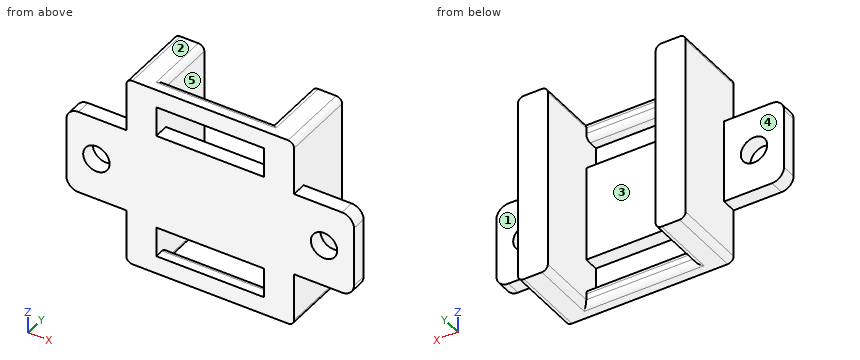
from build123d import *

# Parameters (mm, degrees)
SKETCH1_W           = 28
SKETCH1_H           = 32
BOSS_EXTRUDE1_DEPTH = 2.5
BOSS_EXTRUDE3_DEPTH = 10
SKETCH3_W           = 18
SKETCH3_H           = 8
CUT_EXTRUDE1_DEPTH  = 2.5
SKETCH4_W           = 10
SKETCH4_H           = 14
SKETCH4_R           = 2.2
BOSS_EXTRUDE4_DEPTH = 2.5
FILLET1_R           = 2
FILLET2_R           = 1
SKETCH5_W           = 24.202572411
SKETCH5_H           = 3
SKETCH5_W_2         = 23.282926667
BOSS_EXTRUDE5_DEPTH = 2.5
FILLET3_R           = 1


with BuildPart() as part:
    # Sketch1 → Boss-Extrude1 (new body)
    with BuildSketch(Plane(origin=(0, 0, 0), x_dir=(1, 0, 0), z_dir=(0, 1, 0))):
        with Locations((14, 16)):
            Rectangle(SKETCH1_W, SKETCH1_H)
    extrude(amount=BOSS_EXTRUDE1_DEPTH)

    # Sketch2 → Boss-Extrude3 (add)
    with BuildSketch(Plane(origin=(0, 2.5, 0), x_dir=(1, 0, 0), z_dir=(0, 1, 0))):
        Polygon((0, 32), (5, 32), (5, 30), (5, 0), (0, 0), align=None)
        Polygon((28, 0), (23, 0), (23, 30), (23, 32), (28, 32), align=None)
    extrude(amount=BOSS_EXTRUDE3_DEPTH)

    # Sketch3 → Cut-Extrude1 (cut)
    with BuildSketch(Plane(origin=(0, 2.5, 0), x_dir=(1, 0, 0), z_dir=(0, 1, 0))):
        with Locations((14, 28)):
            Rectangle(SKETCH3_W, SKETCH3_H)
        with Locations((14, 4)):
            Rectangle(SKETCH3_W, SKETCH3_H)
    extrude(amount=-CUT_EXTRUDE1_DEPTH, mode=Mode.SUBTRACT)

    # Sketch4 → Boss-Extrude4 (add)
    # profile 1 of 2: a face of its own
    with BuildSketch(Plane.XZ):
        with Locations((-5, -16)):
            Rectangle(SKETCH4_W, SKETCH4_H)
        with Locations(Location((-5, -16, 0), (0, 0, 270))):
            Circle(SKETCH4_R, mode=Mode.SUBTRACT)
    # profile 2 of 2: a face of its own
    with BuildSketch(Plane.XZ):
        with Locations((33, -16)):
            Rectangle(SKETCH4_W, SKETCH4_H)
        with Locations(Location((33, -16, 0), (0, 0, 270))):
            Circle(SKETCH4_R, mode=Mode.SUBTRACT)
    extrude(amount=-BOSS_EXTRUDE4_DEPTH)

    # Fillet1
    fillet1_edges = [part.edges().sort_by_distance(p)[0] for p in [
        (-10, 1.25, -23),
        (-10, 1.25, -9),
        (38, 1.25, -9),
        (38, 1.25, -23),
    ]]
    fillet(fillet1_edges, radius=FILLET1_R)

    # Fillet2
    fillet2_edges = [part.edges().sort_by_distance(p)[0] for p in [
        (23, 6.25, -32),
        (23, 6.25, 0),
        (5, 6.25, 0),
        (5, 6.25, -32),
        (0, 6.25, -32),
        (28, 6.25, -32),
        (28, 6.25, 0),
        (0, 6.25, 0),
    ]]
    fillet(fillet2_edges, radius=FILLET2_R)

    # Sketch5 → Boss-Extrude5 (add)
    with BuildSketch(Plane.XZ):
        with Locations((14.601286206, -1.5)):
            Rectangle(SKETCH5_W, SKETCH5_H)
        with Locations((14.141463334, -30.5)):
            Rectangle(SKETCH5_W_2, SKETCH5_H)
    extrude(amount=-BOSS_EXTRUDE5_DEPTH)

    # Fillet3
    fillet3_edges = [part.edges().sort_by_distance(p)[0] for p in [
        (14, 2.5, -3),
        (14, 2.5, 0),
        (14, 2.5, -32),
        (14, 2.5, -29),
    ]]
    fillet(fillet3_edges, radius=FILLET3_R)


solid = part.part
Geometry: final body of the model. Coordinates: model frame, mm. Face numbers are marked on the shaded views. A direction names the side the tool comes from. Give positions to 0.01 mm unless a question says otherwise; leave off trailing zeros. Loops run counter-clockwise (first coordinate to the right, second up) from the corner with the lowest first, then second, coordinate; pieces in that order, holes last. Notation, with made-up numbers: (80.5, -37) - (112.5, -37) arc R5 ccw to (112.5, -28) - close; hole circle Ø10 at (-25, 43.25). An arc over 180 degrees is marked (long way). Answer as CSV lines item,"result". Start each with the question number.
1. Section B-B, the plane y = 3.25. Return loops of the section in (x, z).
2. Section D-D, the plane z = -7. Return loops of the section in (x, y).
3. Section A-A, the plane z = -16. Return loops of the section in (x, y).
4. Section C-C, the plane x = 33. Return loops of the section in (y, z), plus the area to 3 significant figures.
5. Reachability of the marked faces 1 and 2 from +Z, -Z, +X, -X, +Y, -Y: full face, straight path, thin tool, end or side. Return the list, or none.
6. Ray query, L1, parallel to X at y = 1.4, z = -16; L2, parallel to X at y = 11.25, z = -19; L3, parallel to Y at x = -2.5, z = -22. Return the intervals inside material, ascending.
7. Draft query along X for the marked faces 3, 4 and 5. Return one class per face: released by +X, released by -X, zero draft, split by the parting line, or undercut.
8. Pin query (flat end, axial travel): P1, Ø1.5, axis at y = 11, z = -7.5, coming from the -X side; P2, Ø0.5, axis at x = 18.5, z = -30.5, coming from the +Y side; P3, Ø3, axis at x = -2.5, y = 1, coming from the -Z side; P4, Ø8, axis at x = 20.5, z = -11.5, coming from the -Y side. Return the tip coordinate at first contact, or that it passes through.
Answers:
1,outline,"(0, -31) arc R1 ccw to (1, -32) - (4, -32) arc R1 ccw to (5, -31) - (5, -1) arc R1 ccw to (4, 0) - (1, 0) arc R1 ccw to (0, -1) - close; (23, -31) arc R1 ccw to (24, -32) - (27, -32) arc R1 ccw to (28, -31) - (28, -1) arc R1 ccw to (27, 0) - (24, 0) arc R1 ccw to (23, -1) - close"
2,outline,"(0, 0) - (5, 0) - (5, 12.5) - (0, 12.5) - close; (23, 0) - (28, 0) - (28, 12.5) - (23, 12.5) - close"
3,outline,"(-10, 0) - (-7.2, 0) - (-7.2, 2.5) - (-10, 2.5) - close; (-2.8, 0) - (30.8, 0) - (30.8, 2.5) - (28, 2.5) - (28, 12.5) - (23, 12.5) - (23, 2.5) - (5, 2.5) - (5, 12.5) - (0, 12.5) - (0, 2.5) - (-2.8, 2.5) - close; (35.2, 0) - (38, 0) - (38, 2.5) - (35.2, 2.5) - close"
4,outline,"(0, -23) - (2.5, -23) - (2.5, -18.2) - (0, -18.2) - close; (0, -13.8) - (2.5, -13.8) - (2.5, -9) - (0, -9) - close"
4,area,"24.0 mm2"
5,face 1,"+Z, -Z, +X, +Y"
5,face 2,"+Z, +X, -X, +Y, -Y"
6,L1,"x = -10 to -7.2, -2.8 to 30.8, 35.2 to 38"
6,L2,"x = 0 to 5, 23 to 28"
6,L3,"y = 0 to 2.5"
7,face 3,"undercut"
7,face 4,"zero draft"
7,face 5,"undercut"
8,P1,"stops at x = 0"
8,P2,"stops at y = 2.5"
8,P3,"stops at z = -23"
8,P4,"stops at y = 0"
